Build history of the part. All positions in model axes, mm. A direction names the side the tool comes from. Round coordinates to 2 decimals unless told otherwise and drop trailing zeros. Write each loop counter-clockwise with the first axis right and the second up, starting at its lowest first coordinate (ties: lowest second). Pieces come first, ordered by that corner, then holes. Notation, with made-up numbers: (29.25, 41.25) -> (52.25, 41.25) arc R15 ccw to (52.25, 64.25) -> close; hole circle Ø2 at (63, 37.5). An arc over 180 degrees is marked (long way). Answer in a Markdown table with one row per item.
```python
from build123d import *

# Parameters (mm, degrees)
SKETCH_1_W             = 60
SKETCH_1_H             = 65
EXTRUDE_1_DEPTH        = 60
SKETCH_2_W             = 60
SKETCH_2_H             = 55
CUT_EXTRUDE_1_DEPTH    = 50
CUT_EXTRUDE_2_DEPTH    = 61
HOLE_WIZARD_M3_1_D     = 2.5
HOLE_WIZARD_M3_1_DEPTH = 7.5
HOLE_WIZARD_M3_1_TIP   = 0.751075774


with BuildPart() as part:
    # 草图1 → 凸台-拉伸1 (new body)
    with BuildSketch(Plane.XY):
        Rectangle(SKETCH_1_W, SKETCH_1_H)
    extrude(amount=EXTRUDE_1_DEPTH)

    # 草图2 → 切除-拉伸1 (cut)
    with BuildSketch(Plane(origin=(0, 0, 0), x_dir=(-1, 0, 0), z_dir=(0, 0, -1))):
        with Locations((0, -5)):
            Rectangle(SKETCH_2_W, SKETCH_2_H)
    extrude(amount=-CUT_EXTRUDE_1_DEPTH, mode=Mode.SUBTRACT)

    # 草图3 → 切除-拉伸2 (cut, through all)
    with BuildSketch(Plane.XY.offset(60)):
        with BuildLine():
            Line((-23.2, -22.5), (-23.2, -16.5))
            ThreePointArc((-23.2, -16.5), (-20, -13.3), (-16.8, -16.5))
            Line((-16.8, -16.5), (-16.8, -22.5))
            ThreePointArc((-16.8, -22.5), (-20, -25.7), (-23.2, -22.5))
        make_face()
        with BuildLine():
            Line((23.2, -22.5), (23.2, -16.5))
            ThreePointArc((23.2, -16.5), (20, -13.3), (16.8, -16.5))
            Line((16.8, -16.5), (16.8, -22.5))
            ThreePointArc((16.8, -22.5), (20, -25.7), (23.2, -22.5))
        make_face()
    extrude(amount=-CUT_EXTRUDE_2_DEPTH, mode=Mode.SUBTRACT)

    # M3 螺纹孔1
    with Locations(Plane(origin=(0, 32.5, 10), x_dir=(1, 0, 0), z_dir=(0, 1, 0))):
        with Locations((0, 0), (0, -40)):
            Hole(HOLE_WIZARD_M3_1_D / 2, depth=HOLE_WIZARD_M3_1_DEPTH)
            with Locations((0, 0, -(HOLE_WIZARD_M3_1_DEPTH + HOLE_WIZARD_M3_1_TIP / 2))):  # 118° drill point
                Cone(0, HOLE_WIZARD_M3_1_D / 2, HOLE_WIZARD_M3_1_TIP, mode=Mode.SUBTRACT)


solid = part.part
```
Q1. Drop flat-ended pins along their axis: P1, Ø2, axis at x = 0, z = 10, coming from the -Y side; P2, Ø10, axis at x = 3.5, y = 13.5, coming from the -Z side. Give the stop position or say it passes through.
A:
| item | result |
|---|---|
| P1 | y = 22.5 |
| P2 | z = 50 |
Q2. Saw through at D-D on z = 33. Write the cut outline in (x, y), plus the area to 3 significant figures.
A:
| item | result |
|---|---|
| outline | (-30, 22.5) -> (30, 22.5) -> (30, 32.5) -> (-30, 32.5) -> close |
| area | 600 mm² |
Q3. Two-plate mould, pull along X, no slides. Class faces 1 (the flat face through (-30, 9, 52)), 2 (the flat face through (-16.8, -19, 55)), 3 (the flat face through (0, -32.5, 55)): released by +X, released by -X, zero draft, split by the parting line, or undercut.
A:
| item | result |
|---|---|
| face 1 | released by -X |
| face 2 | undercut |
| face 3 | zero draft |
Q4. Saw through at A-A on x = -20. Write the cut outline in (y, z), plus the area to 3 significant figures.
A:
| item | result |
|---|---|
| outline | (-32.5, 50) -> (-25.7, 50) -> (-25.7, 60) -> (-32.5, 60) -> close; (-13.3, 50) -> (22.5, 50) -> (22.5, 0) -> (32.5, 0) -> (32.5, 60) -> (-13.3, 60) -> close |
| area | 1,030 mm² |
Q5. Which spindle directions (+Z, -Z, +X, -X, +Y, -Y) get a long thin tool onto all of the face, cutting with end or side? Do faces 4 (the flat face through (0, -5, 50)), 5 (the flat face through (16.8, -19, 55)), 6 (the cylindrical face through (0.16, 28.7, 48.76)). Say none if no direction does.
A:
| item | result |
|---|---|
| face 4 | -Z, +X, -X, -Y |
| face 5 | +Z, -Z |
| face 6 | +Y |
Q6. Saw through at B-B on z = 53. Write the cut outline in (x, y).
A:
| item | result |
|---|---|
| outline | (-30, -32.5) -> (30, -32.5) -> (30, 32.5) -> (-30, 32.5) -> close; hole (-23.2, -22.5) arc R3.2 ccw to (-16.8, -22.5) -> (-16.8, -16.5) arc R3.2 ccw to (-23.2, -16.5) -> close; hole (16.8, -22.5) arc R3.2 ccw to (23.2, -22.5) -> (23.2, -16.5) arc R3.2 ccw to (16.8, -16.5) -> close |
Q7. Saw through at C-C on y = -18. Write the cut outline in (x, z).
A:
| item | result |
|---|---|
| outline | (-30, 50) -> (-23.2, 50) -> (-23.2, 60) -> (-30, 60) -> close; (-16.8, 50) -> (16.8, 50) -> (16.8, 60) -> (-16.8, 60) -> close; (23.2, 50) -> (30, 50) -> (30, 60) -> (23.2, 60) -> close |
Q8. Wall check: line 1 (Z direction, x = 0, y = 30); line 2 (X direction, y = 30.75, z = 50); line 3 (Y direction, x = 17.5, z = 43.5). Give the ranges that are in metal, low to high. Write a range as [from, to].
A:
| item | result |
|---|---|
| line 1 | [0, 8.75], [11.25, 48.75], [51.25, 60] |
| line 2 | [-30, -1.25], [1.25, 30] |
| line 3 | [22.5, 32.5] |
